Autodesk Inventor part; units mm, degrees
ref_plane "YZ Plane" through (0, 0, 0) normal (1, 0, 0) x (0, 1, 0)
ref_plane "XZ Plane" through (0, 0, 0) normal (0, 1, 0) x (-1, 0, 0)
ref_plane "XY Plane" through (0, 0, 0) normal (0, 0, 1) x (1, 0, 0)
sketch "Sketch1" plane through (0, 0, 0) normal (0, 1, 0) x (-1, 0, 0)
  circle A0 centre (0, 0) radius 2.95
  dimension "d0" = 5.9
extrude "Extrusion1" add sketch "Sketch1" along normal blind 9
sketch "Sketch2" plane through (0, 9, 0) normal (0, 1, 0) x (1, 0, 0)
  circle A0 centre (0, 0) radius 5
  circle A1 centre (0, 0) radius 3
  dimension "d3" = 10
  dimension "d6" = 6
extrude "Extrusion2" add sketch "Sketch2" along normal blind 25 contours A0 | A1
sketch "Sketch3" plane through (0, 34, 0) normal (0, 1, 0) x (1, 0, 0)
  circle A0 centre (0, 0) radius 2.95
  circle A1 centre (0, 0) radius 2.95
  dimension "d7" = 5.9
extrude "Extrusion3" add sketch "Sketch3" along normal blind 9
properties part number "Peg"
Check sheet for the modelled part. Datum: model origin and axes. Units: mm. A direction names the side the tool comes from. Round coordinates to 2 decimals unless told otherwise and drop trailing zeros. Loops run counter-clockwise (first coordinate to the right, second up) from the corner with the lowest first, then second, coordinate; pieces in that order, holes last.
1. Set-up check for faces 1 (the cylindrical face through (2.947, 4.437, -0.13)), 2 (the flat face through (0, 43, 0)), 3 (the cylindrical face through (-2.947, 38.437, 0.13)): record each of +Z, -Z, +X, -X, +Y, -Y from which the full face is reachable in a straight line by a thin tool's end or side.
2. Sectioned sample at B-B on z = 0. Record the boundary of the cut face in (x, y), and give its area (3 significant figures).
3. Gauge pin test, flat end, axial feed: pin 1 Ø2 at (x, z) = (-4, 3.5) entering from -Y. Record the tip position at first contact, or that the pin passes through.
4. Sectioned sample at C-C on y = 22.5. Record the boundary of the cut face in (x, z).
5. Sectioned sample at D-D on y = 40. Record the boundary of the cut face in (x, z).
6. Sectioned sample at A-A on x = 0. Record the boundary of the cut face in (y, z), and give its area (3 significant figures).
7. Scan lines: probe 1 along Y at (x, z) = (-3.5, 0); probe 2 along X at (y, z) = (25.5, 4.25); probe 3 along Z at (x, y) = (2.25, 34.5). Record each from-to range of solid material in increasing order.
Recorded:
1. face 1: -Y
1. face 2: +Z, -Z, +X, -X, +Y
1. face 3: +Y
2. outline: (-5, 9) - (-2.95, 9) - (-2.95, 0) - (2.95, 0) - (2.95, 9) - (5, 9) - (5, 34) - (2.95, 34) - (2.95, 43) - (-2.95, 43) - (-2.95, 34) - (-5, 34) - close
2. area: 356 mm2
3. pin 1: stops at y = 9
4. outline: circle Ø10 at (0, 0)
5. outline: circle Ø5.9 at (0, 0)
6. outline: (0, -2.95) - (9, -2.95) - (9, -5) - (34, -5) - (34, -2.95) - (43, -2.95) - (43, 2.95) - (34, 2.95) - (34, 5) - (9, 5) - (9, 2.95) - (0, 2.95) - close
6. area: 356 mm2
7. probe 1: y = 9 to 34
7. probe 2: x = -2.63 to 2.63
7. probe 3: z = -1.91 to 1.91
